Can you work these out from the drawing? Everything is in mm from the part's minimum corner. A direction names the side the tool comes from. Give positions to 0.01 mm unless a question says otherwise; leave off trailing zeros. Write each loop counter-clockwise with the first axis right and the second up, starting at its lowest first coordinate (ties: lowest second). Pieces come first, ordered by that corner, then holes. Notation, with made-up numbers: (62.5, 32) - (72.5, 32) arc R17 cw to (72.5, 62) - close; hole circle Ø10 at (35, 64.25). An arc over 180 degrees is marked (long way). Use a Markdown table: item, result.
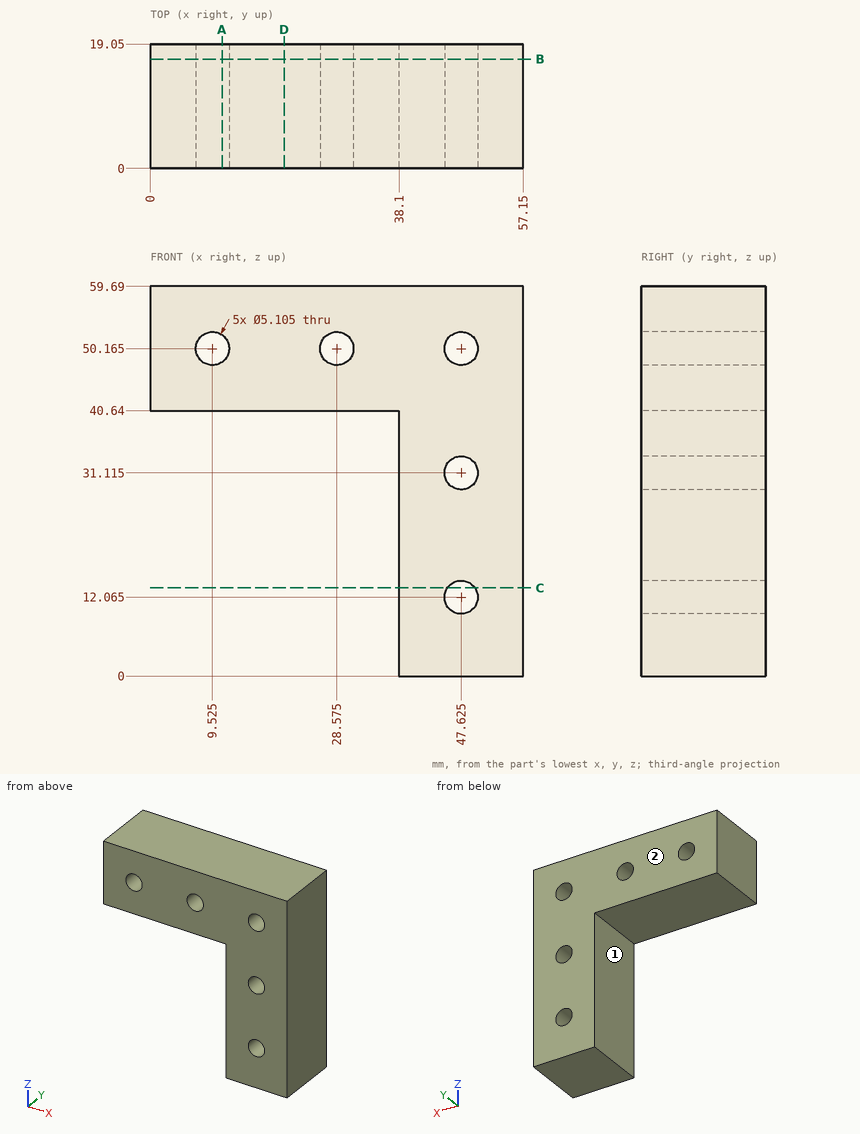
Item 1: Will these pins go through, and if not, where does the flat tip stop? pin 1 Ø6 at (x, y) = (15.5, 15.5) entering from -Z; pin 2 Ø10 at (y, z) = (4.5, 13) entering from -X.
Values:
| item | result |
|---|---|
| pin 1 | stops at z = 40.64 |
| pin 2 | stops at x = 38.1 |
Item 2: For the marked faces 1 and 2, which set-ups out of +Z, -Z, +X, -X, +Y, -Y let a thin tool reach every point of the face, with its end or its side?
Values:
| item | result |
|---|---|
| face 1 | -Z, -X, +Y, -Y |
| face 2 | +Z, -Z, +X, -X, +Y |
Item 3: I need wall thicknesses on line 1 along X through (y, z) = (17.5, 12); line 2 along X through (y, z) = (8.5, 20.5); line 3 along X through (y, z) = (1.5, 32). Which ranges of each line are inside material? Lowest first, please. Write a range as [from, to].
Values:
| item | result |
|---|---|
| line 1 | x = [38.1, 45.07], [50.18, 57.15] |
| line 2 | x = [38.1, 57.15] |
| line 3 | x = [38.1, 45.23], [50.02, 57.15] |
Item 4: If we section it at A-A, the plane x = 11: Write out the boundary of the cut face in (y, z).
Values:
| item | result |
|---|---|
| outline | (0, 40.64) - (19.05, 40.64) - (19.05, 48.08) - (0, 48.08) - close; (0, 52.25) - (19.05, 52.25) - (19.05, 59.69) - (0, 59.69) - close |
Item 5: If we section it at C-C, the plane z = 13.5: Write out the boundary of the cut face in (x, y).
Values:
| item | result |
|---|---|
| outline | (38.1, 0) - (45.51, 0) - (45.51, 19.05) - (38.1, 19.05) - close; (49.74, 0) - (57.15, 0) - (57.15, 19.05) - (49.74, 19.05) - close |
Item 6: If we section it at B-B, the plane y = 16.75: Count the separate pieces of the cut face and the enclosed holes in it, plus the area to 3 significant figures.
Values:
| item | result |
|---|---|
| separate pieces | 1 |
| enclosed holes | 5 |
| area | 1,760 mm2 |
Item 7: If we section it at D-D, the plane x = 20.5: Write out the boundary of the cut face in (y, z).
Values:
| item | result |
|---|---|
| outline | (0, 40.64) - (19.05, 40.64) - (19.05, 59.69) - (0, 59.69) - close |
